from build123d import *

# Parameters (mm, degrees)
SKETCH1_W           = 420
SKETCH1_H           = 320
SKETCH1_W_2         = 400
SKETCH1_H_2         = 300
BOSS_EXTRUDE1_DEPTH = 250
SKETCH2_W           = 420
SKETCH2_H           = 320
BOSS_EXTRUDE2_DEPTH = 10


with BuildPart() as part:
    # Sketch1 → Boss-Extrude1 (new body)
    with BuildSketch(Plane.XY):
        with Locations((200, -150)):
            Rectangle(SKETCH1_W, SKETCH1_H)
        with Locations((200, -150)):
            Rectangle(SKETCH1_W_2, SKETCH1_H_2, mode=Mode.SUBTRACT)
    extrude(amount=BOSS_EXTRUDE1_DEPTH)

    # Sketch2 → Boss-Extrude2 (add)
    with BuildSketch(Plane.XY.offset(250)):
        with Locations((200, -150)):
            Rectangle(SKETCH2_W, SKETCH2_H)
    extrude(amount=BOSS_EXTRUDE2_DEPTH)


solid = part.part
The model under review builds one solid part; all positions refer to its coordinate system, in mm. A direction names the side the tool comes from. Round coordinates to 2 decimals unless told otherwise and drop trailing zeros. Write each loop counter-clockwise with the first axis right and the second up, starting at its lowest first coordinate (ties: lowest second). Pieces come first, ordered by that corner, then holes. Notation, with made-up numbers: M 67.25,42 L 95.25,42 A18 cw 95.25,73 Z; hole C 65,-13 d3. An arc over 180 degrees is marked long. Use a Markdown table: item, result. Add a question column.
Q1. We need section A-A, the plane z = 85. State the section outline as (x, y) points.
Q2. We need section B-B, the plane y = -255. State the section outline as (x, z) points.
Q3. The part is to be moulded in two halves that separate along X. For faces 3 (the face through (197, -148, 260)), 4 (the face through (197, -300, 123)), 5 (the face through (-10, -152, 128)), say which applies: pulls with the +X half, pulls with the -X half, needs draft (parallel to the pull), parting line crosses it, or undercut.
Q4. To check wall thickness, follow line 1 (Y direction, x = 153, z = 229); line 2 (X direction, y = -180, z = 88); line 3 (Z direction, x = 222.5, y = -193.5). State the ranges of each line that lie inside material, in increasing order.
Q5. Machinability: for faces 1 (the face through (197, 0, 123)), 2 (the face through (197, 10, 128)), which of the approach directions +Z, -Z, +X, -X, +Y, -Y give a long, thin tool a straight path to every point of the face, cutting with its end or side? Answer none if there is none.
Q6. We need section C-C, the plane x = 105. State the section outline as (y, z) points.
Q7. Insertion check: pin 1 (2 mm diameter, centred on x = 324, y = -129, fed in from -Z). The pin has a flat end and moves straight along its axis. Give the tip position at first contact, or say it passes through.
Findings below:
| question | item | result |
|---|---|---|
| 1 | outline | M -10,-310 L 410,-310 L 410,10 L -10,10 Z; hole M 0,-300 L 400,-300 L 400,0 L 0,0 Z |
| 2 | outline | M -10,0 L 0,0 L 0,250 L 400,250 L 400,0 L 410,0 L 410,260 L -10,260 Z |
| 3 | face 3 | needs draft |
| 3 | face 4 | undercut |
| 3 | face 5 | pulls with the -X half |
| 4 | line 1 | y = -310 to -300, 0 to 10 |
| 4 | line 2 | x = -10 to 0, 400 to 410 |
| 4 | line 3 | z = 250 to 260 |
| 5 | face 1 | -Z |
| 5 | face 2 | +Z, -Z, +X, -X, +Y |
| 6 | outline | M -310,0 L -300,0 L -300,250 L 0,250 L 0,0 L 10,0 L 10,260 L -310,260 Z |
| 7 | pin 1 | stops at z = 250 |
